```python
from build123d import *

# Parameters (mm, degrees)
F0_W        = 69.85
F0_H        = 88.9
F1_DEPTH    = 63.5
F2_T        = -2.54
F0_H_2      = 19.05
F3_DEPTH    = 63.5
F4_T        = 2.54
F4_T3_DEPTH = 91.44
F4_T5_DEPTH = 69.85
F4_T7_DEPTH = 63.5


# Not quite as in the source:
# - a shell that OpenCascade refuses in one call is made with other operations: the cavity is built on its own and cut out


with BuildPart() as f1:
    # F0 (on Front) → F1 (new body)
    with BuildSketch(Plane.XZ):
        with Locations((-9.7199578146, -2.0941891145)):
            Rectangle(F0_W, F0_H)
    extrude(amount=F1_DEPTH)

    # F2
    f2_openings = [f1.faces().sort_by_distance(p)[0] for p in [
        (-9.719958, -31.75, 42.355811),
    ]]
    offset(amount=F2_T, openings=f2_openings)

    # F0 (on Front) → F3 (join)
    with BuildSketch(Plane.XZ):
        with Locations((-9.7199578146, -56.0691891145)):
            Rectangle(F0_W, F0_H_2)
    extrude(amount=F3_DEPTH)

    # F4: shell of thickness 2.54, made by hand


with BuildPart() as f4_core1:
    # F4_t2: copy of F1
    add(f1.part)

    # the walls: a layer under each face that stays
    f4_faces = [f4_core1.faces().sort_by_distance(p)[0] for p in [
        (-44.6449578146, -31.75, -11.6191891145),
        (-9.7199578146, 0, -11.6191891145),
        (25.2050421854, -31.75, -11.6191891145),
        (-9.7199578146, -31.75, -65.5941891145),
        (22.8767088521, -61.3833333333, 42.3558108855),
        (-9.7199578146, -60.96, -0.8241891145),
        (-9.7199578146, -31.75, -44.0041891145),
        (-42.1049578146, -31.75, -0.8241891145),
        (-9.7199578146, -2.54, -0.8241891145),
        (22.6650421854, -31.75, -0.8241891145),
    ]]
    thicken(f4_faces, amount=-F4_T, mode=Mode.SUBTRACT)

    # F4_s4 → F4_t3 (cut)
    with BuildSketch(Plane.XY.offset(-46.5441891145)):
        Polygon((-42.0795578146, -60.9346), (-42.1049578146, -63.5), (-44.6449578146, -63.5), (-44.6449578146, -60.96), align=None)
        Polygon((22.6396421854, -60.9346), (22.6650421854, -63.5), (25.2050421854, -63.5), (25.2050421854, -60.96), align=None)
        Polygon((-42.0795578146, -2.5654), (-44.6449578146, -2.54), (-44.6449578146, 0), (-42.1049578146, 0), align=None)
        Polygon((22.6396421854, -2.5654), (22.6650421854, 0), (25.2050421854, 0), (25.2050421854, -2.54), align=None)
    extrude(amount=F4_T3_DEPTH, mode=Mode.SUBTRACT)

    # F4_s6 → F4_t5 (cut)
    with BuildSketch(Plane.YZ.offset(-44.6449578146)):
        Polygon((-60.9346, -43.9787891145), (-63.5, -44.0041891145), (-63.5, -46.5441891145), (-60.96, -46.5441891145), align=None)
        Polygon((-2.5654, -43.9787891145), (-2.54, -46.5441891145), (0, -46.5441891145), (0, -44.0041891145), align=None)
    extrude(amount=F4_T5_DEPTH, mode=Mode.SUBTRACT)

    # F4_s8 → F4_t7 (cut)
    with BuildSketch(Plane.XZ):
        Polygon((22.6396421854, -43.9787891145), (22.6650421854, -46.5441891145), (25.2050421854, -46.5441891145), (25.2050421854, -44.0041891145), align=None)
        Polygon((-42.0795578146, -43.9787891145), (-42.1049578146, -46.5441891145), (-44.6449578146, -46.5441891145), (-44.6449578146, -44.0041891145), align=None)
    extrude(amount=F4_T7_DEPTH, mode=Mode.SUBTRACT)


with BuildPart() as f1_1:
    add(f1.part)

    # what is left inside the walls is the cavity
    f4_cavity = [f4_core1.part.solids().sort_by_distance(p)[0] for p in [
        (-9.719958, -43.18, -63.028789),
    ]]
    add(f4_cavity, mode=Mode.SUBTRACT)


solid = f1_1.part
```
Can you work these out from the model? Positions are in its coordinate system, mm. A direction names the side the tool comes from. Round coordinates to 2 decimals unless told otherwise and drop trailing zeros. Loops run counter-clockwise (first coordinate to the right, second up) from the corner with the lowest first, then second, coordinate; pieces in that order, holes last.
Item 1: Please list where these lines run through material, in increasing order: L1, parallel to Y at x = -13, z = -6.5; L2, parallel to Z at x = -30, y = -51; L3, parallel to X at y = -60, z = 24.5.
Item 2: Suppose I cut it at C-C, the plane x = 14. Write out the boundary of the cut face in (y, z), then the cut area to 3 significant figures.
Item 3: Suppose I cut it at B-B, the plane z = -18. Write out the boundary of the cut face in (x, y).
Item 4: Which directions (+Z, -Z, +X, -X, +Y, -Y) give clear straight access to the entire face, cutting with the end or side of a thin tool? Please do faces 1 (the flat face through (-10, -33, -63.054)), 2 (the flat face through (22.665, -31, -1)), 3 (the flat face through (-10, -63.5, 1)).
Item 5: Will these pins go through, and if not, where does the flat tip stop? pin 1 Ø5 at (x, z) = (-24.5, -57.5) entering from -Y; pin 2 Ø1 at (x, y) = (-24.5, -19.5) entering from +Z.
Item 6: Suppose I cut it at A-A, the plane y = -24. Write out the boundary of the cut face in (x, z).
Item 7: If we mould it in two halves opening along Z, with no side actions, what happens to faces 4 (the flat face through (-10, -31, -44.004)), 5 (the flat face through (22.665, -33, -55)), 6 (the flat face through (-10, -31, -65.594))? For each: +Z half, -Z half, draft (parallel to the pull), parting line (faces both ways), or undercut.
Reported:
1. L1: y = -63.5 to -60.96, -2.54 to 0
1. L2: z = -65.59 to -63.05, -46.54 to -44
1. L3: x = -44.64 to -42.1, 22.67 to 25.21
2. outline: (-63.5, -65.59) - (0, -65.59) - (0, 42.36) - (-2.54, 42.36) - (-2.54, -44) - (-60.96, -44) - (-60.96, 42.36) - (-63.5, 42.36) - (-63.5, -46.54) - (-2.54, -46.54) - (-2.54, -63.05) - (-63.5, -63.05) - close
2. area: 803 mm2
3. outline: (-44.64, -63.5) - (25.21, -63.5) - (25.21, 0) - (-44.64, 0) - close; hole (-42.1, -60.96) - (22.67, -60.96) - (22.67, -2.54) - (-42.1, -2.54) - close
4. face 1: -Y
4. face 2: +Z
4. face 3: +Z, -Z, +X, -X, -Y
5. pin 1: stops at y = -2.54
5. pin 2: stops at z = -44
6. outline: (-44.64, -65.59) - (25.21, -65.59) - (25.21, 42.36) - (22.67, 42.36) - (22.67, -44) - (-42.1, -44) - (-42.1, 42.36) - (-44.64, 42.36) - close; hole (-42.1, -63.05) - (22.67, -63.05) - (22.67, -46.54) - (-42.1, -46.54) - close
7. face 4: +Z half
7. face 5: undercut
7. face 6: -Z half
